from build123d import *

# Parameters (mm, degrees)
RESSALTO_EXTRUS_O1_DEPTH = 3


with BuildPart() as part:
    # Esboço1 → Ressalto-extrusão1 (new body)
    with BuildSketch(Plane(origin=(0, 0, 0), x_dir=(0, 0, -1), z_dir=(1, 0, 0))):
        Polygon((9.606615439, 38.402396467), (-6.893384561, 38.402396467), (-6.893384561, 41.402396467), (-14.893384561, 41.402396467), (-14.893384561, 38.402396467), (-14.893384561, 1.302396467), (-14.893384561, -1.697603533), (-6.893384561, -1.697603533), (-6.893384561, 1.302396467), (9.606615439, 1.302396467), (10.106615439, 1.302396467), (12.106615439, 1.302396467), (12.606615439, 1.302396467), (12.606615439, 6.302396467), (11.231615439, 6.302396467), (11.231615439, 8.802396467), (12.606615439, 8.802396467), (12.606615439, 14.302396467), (15.606615439, 14.302396467), (15.606615439, 8.802396467), (16.981615439, 8.802396467), (16.981615439, 6.302396467), (15.606615439, 6.302396467), (15.606615439, 1.302396467), (18.106615439, 1.302396467), (18.106615439, 38.402396467), (15.606615439, 38.402396467), (15.606615439, 33.402396467), (16.981615439, 33.402396467), (16.981615439, 30.902396467), (15.606615439, 30.902396467), (15.606615439, 25.402396467), (12.606615439, 25.402396467), (12.606615439, 30.902396467), (11.231615439, 30.902396467), (11.231615439, 33.402396467), (12.606615439, 33.402396467), (12.606615439, 38.402396467), (12.106615439, 38.402396467), (10.106615439, 38.402396467), align=None)
        with BuildLine():
            Line((-7.41891132, 18.243485959), (-1.631744546, 11.928665745))
            ThreePointArc((-1.631744546, 11.928665745), (-1.106217787, 10.577396467), (-1.631744546, 9.226127189))
            Line((-1.631744546, 9.226127189), (-6.298860449, 4.13348013))
            ThreePointArc((-6.298860449, 4.13348013), (-6.967895473, 3.654102179), (-7.77333369, 3.484749408))
            Line((-7.77333369, 3.484749408), (-10.013435432, 3.484749408))
            ThreePointArc((-10.013435432, 3.484749408), (-10.818873649, 3.654102179), (-11.487908673, 4.13348013))
            Line((-11.487908673, 4.13348013), (-11.867857802, 4.54807168))
            ThreePointArc((-11.867857802, 4.54807168), (-12.257378456, 5.174408714), (-12.393384561, 5.899340958))
            Line((-12.393384561, 5.899340958), (-12.393384561, 15.255451976))
            ThreePointArc((-12.393384561, 15.255451976), (-12.257378456, 15.98038422), (-11.867857802, 16.606721254))
            Line((-11.867857802, 16.606721254), (-10.367857802, 18.243485959))
            ThreePointArc((-10.367857802, 18.243485959), (-8.893384561, 18.892216682), (-7.41891132, 18.243485959))
        make_face(mode=Mode.SUBTRACT)
        with BuildLine():
            Line((3.08108868, 6.786133018), (6.106615439, 3.484749408))
            Line((6.106615439, 3.484749408), (-2.893384561, 3.484749408))
            Line((-2.893384561, 3.484749408), (0.132142198, 6.786133018))
            ThreePointArc((0.132142198, 6.786133018), (1.606615439, 7.434863741), (3.08108868, 6.786133018))
        make_face(mode=Mode.SUBTRACT)
        with BuildLine():
            Line((10.106615439, 17.670043526), (10.106615439, 3.484749408))
            Line((10.106615439, 3.484749408), (9.512091327, 4.13348013))
            Line((9.512091327, 4.13348013), (4.844975424, 9.226127189))
            ThreePointArc((4.844975424, 9.226127189), (4.319448665, 10.577396467), (4.844975424, 11.928665745))
            Line((4.844975424, 11.928665745), (10.106615439, 17.670043526))
        make_face(mode=Mode.SUBTRACT)
        with BuildLine():
            ThreePointArc((3.08108868, 14.368659915), (1.606615439, 13.719929193), (0.132142198, 14.368659915))
            Line((0.132142198, 14.368659915), (-3.655024576, 18.501127189))
            ThreePointArc((-3.655024576, 18.501127189), (-4.180551335, 19.852396467), (-3.655024576, 21.203665745))
            Line((-3.655024576, 21.203665745), (0.132142198, 25.336133018))
            ThreePointArc((0.132142198, 25.336133018), (1.606615439, 25.984863741), (3.08108868, 25.336133018))
            Line((3.08108868, 25.336133018), (6.868255454, 21.203665745))
            ThreePointArc((6.868255454, 21.203665745), (7.393782213, 19.852396467), (6.868255454, 18.501127189))
            Line((6.868255454, 18.501127189), (3.08108868, 14.368659915))
        make_face(mode=Mode.SUBTRACT)
        with BuildLine():
            ThreePointArc((-11.867857802, 23.09807168), (-12.257378456, 23.724408714), (-12.393384561, 24.449340958))
            Line((-12.393384561, 24.449340958), (-12.393384561, 33.805451976))
            ThreePointArc((-12.393384561, 33.805451976), (-12.257378456, 34.53038422), (-11.867857802, 35.156721254))
            Line((-11.867857802, 35.156721254), (-11.487908673, 35.571312803))
            ThreePointArc((-11.487908673, 35.571312803), (-10.818873649, 36.050690755), (-10.013435432, 36.220043526))
            Line((-10.013435432, 36.220043526), (-7.77333369, 36.220043526))
            ThreePointArc((-7.77333369, 36.220043526), (-6.967895473, 36.050690755), (-6.298860449, 35.571312803))
            Line((-6.298860449, 35.571312803), (-1.631744546, 30.478665745))
            ThreePointArc((-1.631744546, 30.478665745), (-1.106217787, 29.127396467), (-1.631744546, 27.776127189))
            Line((-1.631744546, 27.776127189), (-7.41891132, 21.461306974))
            ThreePointArc((-7.41891132, 21.461306974), (-8.893384561, 20.812576252), (-10.367857802, 21.461306974))
            Line((-10.367857802, 21.461306974), (-11.867857802, 23.09807168))
        make_face(mode=Mode.SUBTRACT)
        with BuildLine():
            Line((9.512091327, 35.571312803), (10.106615439, 36.220043526))
            Line((10.106615439, 36.220043526), (10.106615439, 22.034749408))
            Line((10.106615439, 22.034749408), (4.844975424, 27.776127189))
            ThreePointArc((4.844975424, 27.776127189), (4.319448665, 29.127396467), (4.844975424, 30.478665745))
            Line((4.844975424, 30.478665745), (9.512091327, 35.571312803))
        make_face(mode=Mode.SUBTRACT)
        with BuildLine():
            Line((0.132142198, 32.918659915), (-2.893384561, 36.220043526))
            Line((-2.893384561, 36.220043526), (6.106615439, 36.220043526))
            Line((6.106615439, 36.220043526), (3.08108868, 32.918659915))
            ThreePointArc((3.08108868, 32.918659915), (1.606615439, 32.269929193), (0.132142198, 32.918659915))
        make_face(mode=Mode.SUBTRACT)
    extrude(amount=RESSALTO_EXTRUS_O1_DEPTH)


solid = part.part
The model under review builds one solid part; all positions refer to its coordinate system, in mm. A direction names the side the tool comes from. Give positions to 0.01 mm unless a question says otherwise; leave off trailing zeros. Loops run counter-clockwise (first coordinate to the right, second up) from the corner with the lowest first, then second, coordinate; pieces in that order, holes last. Notation, with made-up numbers: (-8.5, 38.5) -> (45.5, 38.5) arc R18 cw to (45.5, 59.5) -> close; hole circle Ø2 at (-17, -29.5). An arc over 180 degrees is marked (long way). Write each question's results on one line, items separated by ' | '.
1) Tool access review of faces 1 (the face through (1, 12, -15.607)), 2 (the face through (1.48, 34.52, 12.26)), 3 (the face through (1, 41.402, 11)): name each direction out of +Z, -Z, +X, -X, +Y, -Y from which nothing blocks a thin tool from reaching the whole face with its end or side.
Conclusion:
face 1: +X, -X, -Y | face 2: +X, -X | face 3: +Z, -Z, +X, -X, +Y
2) Take a section at C-C, the plane y = 5. Give the boundary of the cut face in (x, z), plus the area to 3 significant figures.
Conclusion:
outline: (0, -18.11) -> (3, -18.11) -> (3, -15.61) -> (0, -15.61) -> close; (0, -12.61) -> (3, -12.61) -> (3, -10.11) -> (0, -10.11) -> close; (0, -8.72) -> (3, -8.72) -> (3, -4.72) -> (0, -4.72) -> close; (0, 1.5) -> (3, 1.5) -> (3, 5.5) -> (0, 5.5) -> close; (0, 12.18) -> (3, 12.18) -> (3, 14.89) -> (0, 14.89) -> close | area: 47.1 mm^2
3) Draft analysis for pull direction Z (two halves, no side actions). For faces 4 (the face through (1, 30.902, -16)), 5 (the face through (1, 36.22, -2)), 6 (the face through (0, 25, -5)), state which applies: pulls with the +Z half, pulls with the -Z half, needs draft (parallel to the pull), parting line crosses it, or undercut.
Conclusion:
face 4: undercut | face 5: undercut | face 6: needs draft
4) Take a section at A-A, the plane y = 24. Give the boundary of the cut face in (x, z).
Conclusion:
outline: (0, -18.11) -> (3, -18.11) -> (3, -10.11) -> (0, -10.11) -> close; (0, -8.31) -> (3, -8.31) -> (3, -4.31) -> (0, -4.31) -> close; (0, 1.09) -> (3, 1.09) -> (3, 5.09) -> (0, 5.09) -> close; (0, 12.34) -> (3, 12.34) -> (3, 14.89) -> (0, 14.89) -> close
5) Insertion check: pin 1 Ø1.1 at (x, z) = (2, -12) entering from -Y; pin 2 Ø1.2 at (x, z) = (2, -16.5) entering from +Y. Each pin has a flat end and moves straight along its axis. Give the tip position at first contact, or say it passes through.
Conclusion:
pin 1: stops at y = 1.3 | pin 2: stops at y = 38.4
6) Take a section at D-D, the plane x = 0.65. Count the separate pieces of the cut face and the enclosed holes in it, plus the area to 3 significant figures.
Conclusion:
separate pieces: 1 | enclosed holes: 7 | area: 711 mm^2
7) Take a section at B-B, the plane z = -1. Give the boundary of the cut face in (x, y).
Conclusion:
outline: (0, 1.3) -> (3, 1.3) -> (3, 3.48) -> (0, 3.48) -> close; (0, 7.34) -> (3, 7.34) -> (3, 13.81) -> (0, 13.81) -> close; (0, 25.89) -> (3, 25.89) -> (3, 32.36) -> (0, 32.36) -> close; (0, 36.22) -> (3, 36.22) -> (3, 38.4) -> (0, 38.4) -> close
8) For line 1 along Y through (x, z) = (1.05, 9); line 2 along Z through (x, y) = (0.65, 29); line 3 along Z through (x, y) = (2, 35.5), list the stretches that pass through material, from the lowest coordinate up. Write a range as from..to.
Conclusion:
line 1: y = -1.7..3.48, 18.89..20.82, 36.22..41.4 | line 2: z = -18.11..-15.61, -12.61..-10.11, -4.32..1.11, 12.39..14.89 | line 3: z = -18.11..-15.61, -12.61..-10.11, -9.45..-5.45, 2.23..6.23, 11.55..14.89
